For this review, take the finished solid that the model builds, in its own axes (mm). Give positions to 0.01 mm unless a question says otherwise; leave off trailing zeros. Write each loop counter-clockwise with the first axis right and the second up, starting at its lowest first coordinate (ties: lowest second). Pieces come first, ordered by that corner, then holes.
Q1. We need section A-A (z = 78). Write out the cut boundary in (x, y), then the cut area to 3 significant figures.
Q2. For line 1 (Z direction, x = -14.88, y = -0.6) (3 decimals); line 2 (X direction, y = -0.85, z = 117.99); line 3 (X direction, y = -0.1, z = 17.99), list the stretches that pass through material, from the lowest coordinate up.
Q3. Mouldability with a two-part tool opening along Z and no side actions: class faces 1 (the flat face through (-2, -1.5, -2)), 2 (the cylindrical face through (12.8, 0, 12.1)) as released by +Z, released by -Z, zero draft, split by the parting line, or undercut.
Q4. We need section B-B (x = 57). Write out the cut boundary in (y, z) (3 decimals).
Q5. Insertion check: P1, Ø1.5, axis at x = 26, y = 0, coming from the -Z side (3 decimals); P2, Ø0.9, axis at x = 1.5, y = -0.5, coming from the +Z side (3 decimals). Each pin has a flat end and moves straight along its axis. Give the tip position at first contact, or say it passes through.
Q6. We need section D-D (y = 0.9). Write out the cut boundary in (x, z) (3 decimals), then the cut area to 3 significant figures.
Q7. We need section C-C (z = -78.5). Write out the cut boundary in (x, y), then the cut area to 3 significant figures.
```python
from build123d import *

# Parameters (mm, degrees)
SKETCH1_W                   = 225.24
SKETCH1_H                   = 288.07
BOSS_EXTRUDE1_DEPTH         = 1.5
M4_CLEARANCE_HOLE1_D        = 4.5
F_1_4_CLEARANCE_HOLE1_D     = 6.7564
F_1_4_CLEARANCE_HOLE1_DEPTH = 20
F_1_4_CLEARANCE_HOLE1_TIP   = 2.029827343
SKETCH6_W                   = 125.24
SKETCH6_H                   = 80
SKETCH6_W_2                 = 37.51
SKETCH6_H_2                 = 100
CUT_EXTRUDE1_DEPTH          = 183.861547694


with BuildPart() as part:
    # Sketch1 → Boss-Extrude1 (new, symmetric)
    with BuildSketch(Plane(origin=(0, 0, 0), x_dir=(1, 0, 0), z_dir=(0, 1, 0))):
        Rectangle(SKETCH1_W, SKETCH1_H)
    extrude(amount=BOSS_EXTRUDE1_DEPTH, both=True)

    # M4 Clearance Hole1 (through all)
    with Locations(Plane(origin=(0, 1.5, 0), x_dir=(1, 0, 0), z_dir=(0, 1, 0))):
        with Locations((-14.88, -117.99), (-14.88, -17.99), (35.13, -117.99), (35.13, -17.99)):
            Hole(M4_CLEARANCE_HOLE1_D / 2)

    # 1/4 Clearance Hole1
    with Locations(Plane(origin=(0, 1.5, 0), x_dir=(1, 0, 0), z_dir=(0, 1, 0))):
        with Locations((10.125, -10.035)):
            Hole(F_1_4_CLEARANCE_HOLE1_D / 2, depth=F_1_4_CLEARANCE_HOLE1_DEPTH)
            with Locations((0, 0, -(F_1_4_CLEARANCE_HOLE1_DEPTH + F_1_4_CLEARANCE_HOLE1_TIP / 2))):  # 118° drill point
                Cone(0, F_1_4_CLEARANCE_HOLE1_D / 2, F_1_4_CLEARANCE_HOLE1_TIP, mode=Mode.SUBTRACT)

    # Sketch6 → Cut-Extrude1 (cut, through all)
    with BuildSketch(Plane(origin=(0, 1.5, 0), x_dir=(1, 0, 0), z_dir=(0, 1, 0))):
        with Locations((0, 104.035)):
            Rectangle(SKETCH6_W, SKETCH6_H)
        with Locations((10.125, -94.035)):
            Rectangle(SKETCH6_W_2, SKETCH6_H_2)
    extrude(amount=-CUT_EXTRUDE1_DEPTH, mode=Mode.SUBTRACT)


solid = part.part
```
Computed:
1. outline: (-112.62, -1.5) - (-8.63, -1.5) - (-8.63, 1.5) - (-112.62, 1.5) - close; (28.88, -1.5) - (112.62, -1.5) - (112.62, 1.5) - (28.88, 1.5) - close
1. area: 563 mm2
2. line 1: z = -64.035 to 15.74, 20.24 to 115.74, 120.24 to 144.035
2. line 2: x = -112.62 to -17.13, -12.63 to -8.63, 28.88 to 32.88, 37.38 to 112.62
2. line 3: x = -112.62 to -17.13, -12.63 to 32.88, 37.38 to 112.62
3. face 1: zero draft
3. face 2: undercut
4. outline: (-1.5, -64.035) - (1.5, -64.035) - (1.5, 144.035) - (-1.5, 144.035) - close
5. P1: stops at z = -64.035
5. P2: stops at z = 44.035
6. outline: (-112.62, -144.035) - (-62.62, -144.035) - (-62.62, -64.035) - (62.62, -64.035) - (62.62, -144.035) - (112.62, -144.035) - (112.62, 144.035) - (28.88, 144.035) - (28.88, 44.035) - (-8.63, 44.035) - (-8.63, 144.035) - (-112.62, 144.035) - close; hole circle Ø4.5 at (-14.88, 17.99); hole circle Ø4.5 at (-14.88, 117.99); hole circle Ø6.756 at (10.125, 10.035); hole circle Ø4.5 at (35.13, 17.99); hole circle Ø4.5 at (35.13, 117.99)
6. area: 51,000 mm2
7. outline: (-112.62, -1.5) - (-62.62, -1.5) - (-62.62, 1.5) - (-112.62, 1.5) - close; (62.62, -1.5) - (112.62, -1.5) - (112.62, 1.5) - (62.62, 1.5) - close
7. area: 300 mm2
